from build123d import *

# Parameters (mm, degrees)
F0_R     = 63.5
F1_DEPTH = 6.35
F2_R     = 5.0272245411
F3_DEPTH = 25.4
F4_R     = 2.641238627
F5_DEPTH = 25.4


# Not quite as in the source:
# - the program builds the solid bodies; features that only make, move or delete a surface that nothing else refers to are left out


with BuildPart() as f1:
    # F0 (on Top) → F1 (new body)
    with BuildSketch(Plane.XY):
        Circle(F0_R)
    extrude(amount=F1_DEPTH)

    # F2 (on face) → F3 (cut)
    with BuildSketch(Plane.XY.offset(6.35)):
        with Locations((-51.2941852212, -4.8283813521)):
            Circle(F2_R)
        with Locations((-45.7605943084, 24.1383034736)):
            Circle(F2_R)
        with Locations((-29.6111274511, 42.8337752819)):
            Circle(F2_R)
        with Locations((-33.1189669669, 20.5034371465)):
            Circle(F2_R)
        with Locations((-34.8243303597, -1.5672247391)):
            Circle(F2_R)
        with Locations((-34.8841510713, -25.8116889745)):
            Circle(F2_R)
        with Locations((-14.3142268062, -20.1833639294)):
            Circle(F2_R)
        with Locations((-13.4874591604, 1.3800424058)):
            Circle(F2_R)
        with Locations((-14.4421327859, 27.3816790432)):
            Circle(F2_R)
        with Locations((21.6737631708, 36.5187302232)):
            Circle(F2_R)
        with Locations((9.3525275588, 24.7192624956)):
            Circle(F2_R)
        with Locations((8.9998366311, 0.3057096619)):
            Circle(F2_R)
        with Locations((10.3590181097, -22.3385263234)):
            Circle(F2_R)
        with Locations((28.006831184, -38.7023799121)):
            Circle(F2_R)
        with Locations((25.5425348878, -12.7913486212)):
            Circle(F2_R)
        with Locations((25.1072477549, 9.6053304151)):
            Circle(F2_R)
        with Locations((41.9120192528, 22.4314276129)):
            Circle(F2_R)
        with Locations((42.3262864351, -4.6631796286)):
            Circle(F2_R)
        with Locations((41.8376736343, -26.8122982234)):
            Circle(F2_R)
    extrude(amount=-F3_DEPTH, mode=Mode.SUBTRACT)

    # F4 (on face) → F5 (join)
    with BuildSketch(Plane.XY.offset(6.35)):
        with Locations((-43.0771894753, 40.4972620308)):
            Circle(F4_R)
    extrude(amount=F5_DEPTH)


solid = f1.part
Input: part model. Units: mm. Frame: model coordinates. A direction names the side the tool comes from. Coordinates: 2 decimals unless noted, no trailing zeros. Order: outer loops, then holes, each group sorted by start corner. A loop starts at its lowest first (then second) coordinate and runs counter-clockwise, first axis right, second up. Notation, with made-up numbers: M -12.5,-15.75 L 26.5,-15.75 A22 ccw 26.5,0.25 Z; hole C -30,-31.75 d10. An arc over 180 degrees is marked long. One line per question, with ' | ' between items.
Item 1: Section C-C (x = 0). Output: boundary loops of the cut face in (y, z).
Geometry results:
outline: M -63.5,0 L 63.5,0 L 63.5,6.35 L -63.5,6.35 Z
Item 2: Section A-A (y = -36.5). Output: boundary loops of the cut face in (x, z).
Geometry results:
outline: M -51.96,0 L 23.49,0 L 23.49,6.35 L -51.96,6.35 Z; M 32.53,0 L 51.96,0 L 51.96,6.35 L 32.53,6.35 Z
Item 3: Section D-D (z = 22). Output: boundary loops of the cut face in (x, y), then the cut area to 3 significant figures.
Geometry results:
outline: C -43.08,40.5 d5.28 | area: 21.9 mm^2
Item 4: Draft query along X for faces 3 (the flat face through (-43, 41, 31.75)), 4 (the cylindrical face through (-13.77, -61.99, 3.13)), 5 (the cylindrical face through (-17.477, -1.679, 3.219)). Return one class per face: released by +X, released by -X, zero draft, split by the parting line, or undercut.
Geometry results:
face 3: zero draft | face 4: split by the parting line | face 5: undercut
Item 5: Reachability of faces 1 (the cylindrical face through (-40.637, 39.486, 18.872)), 2 (the flat face through (-1, 1, 0)) from +Z, -Z, +X, -X, +Y, -Y: full face, straight path, thin tool, end or side. Return the list, or none.
Geometry results:
face 1: +Z | face 2: -Z, +X, -X, +Y, -Y
Item 6: Pin query (flat end, axial travel): pin 1 (11.5 mm diameter, centred on x = 42.33, y = -4.66, fed in from +Z); pin 2 (10 mm diameter, centred on x = -36, z = 9, fed in from +Y). Return the tip coordinate at first contact, or that it passes through.
Geometry results:
pin 1: stops at z = 6.35 | pin 2: stops at y = 54.99
Item 7: Ray query, line 1 along Y through (x, z) = (39.5, 2.5); line 2 along Y through (x, z) = (13, 5.5); line 3 along X through (y, z) = (-24, 3). Return the intervals inside material, ascending.
Geometry results:
line 1: y = -49.72 to -31.26, -22.36 to -8.82, -0.51 to 18.02, 26.84 to 49.72 | line 2: y = -62.16 to -26.62, -18.06 to -2.74, 3.35 to 21.26, 28.18 to 62.16 | line 3: x = -58.79 to -39.57, -30.19 to -17.59, -11.04 to 5.61, 15.1 to 37.67, 46 to 58.79
Item 8: Section B-B (z = 3). Give the number of separate pieces and of enclosed holes in the cut face, then the cut area to 3 significant figures.
Geometry results:
separate pieces: 1 | enclosed holes: 19 | area: 11,200 mm^2
